For this review, take the finished solid that the model builds, in its own axes (mm). A direction names the side the tool comes from. Round coordinates to 2 decimals unless told otherwise and drop trailing zeros. Write each loop counter-clockwise with the first axis right and the second up, starting at its lowest first coordinate (ties: lowest second). Pieces come first, ordered by that corner, then holes.
from build123d import *

# Parameters (mm, degrees)
SKETCH6_R           = 24
BOSS_EXTRUDE1_DEPTH = 5
SKETCH8_R           = 1.55
CUT_EXTRUDE6_DEPTH  = 5
SKETCH10_R          = 4
BOSS_EXTRUDE2_DEPTH = 36
SKETCH11_R          = 3.5
CUT_EXTRUDE8_DEPTH  = 3


with BuildPart() as part:
    # Sketch6 → Boss-Extrude1 (new body)
    with BuildSketch(Plane.XY):
        Circle(SKETCH6_R)
    extrude(amount=BOSS_EXTRUDE1_DEPTH)

    # Sketch8 → Cut-Extrude6 (cut)
    with BuildSketch(Plane(origin=(0, 0, 0), x_dir=(-1, 0, 0), z_dir=(0, 0, -1))):
        with Locations((0, 20)):
            Circle(SKETCH8_R)
        with Locations((14.142135624, 14.142135624)):
            Circle(SKETCH8_R)
        with Locations((20, 0)):
            Circle(SKETCH8_R)
        with Locations((14.142135624, -14.142135624)):
            Circle(SKETCH8_R)
        with Locations((0, -20)):
            Circle(SKETCH8_R)
        with Locations((-14.142135624, -14.142135624)):
            Circle(SKETCH8_R)
        with Locations((-20, 0)):
            Circle(SKETCH8_R)
        with Locations((-14.142135624, 14.142135624)):
            Circle(SKETCH8_R)
    extrude(amount=-CUT_EXTRUDE6_DEPTH, mode=Mode.SUBTRACT)

    # Sketch10 → Boss-Extrude2 (add)
    with BuildSketch(Plane.XY.offset(5)):
        Circle(SKETCH10_R)
    extrude(amount=BOSS_EXTRUDE2_DEPTH)

    # Sketch11 → Cut-Extrude8 (cut)
    with BuildSketch(Plane.XY.offset(5)):
        with Locations((0, 20)):
            Circle(SKETCH11_R)
        with Locations((14.142135624, 14.142135624)):
            Circle(SKETCH11_R)
        with Locations((20, 0)):
            Circle(SKETCH11_R)
        with Locations((14.142135624, -14.142135624)):
            Circle(SKETCH11_R)
        with Locations((0, -20)):
            Circle(SKETCH11_R)
        with Locations((-14.142135624, -14.142135624)):
            Circle(SKETCH11_R)
        with Locations((-20, 0)):
            Circle(SKETCH11_R)
        with Locations((-14.142135624, 14.142135624)):
            Circle(SKETCH11_R)
    extrude(amount=-CUT_EXTRUDE8_DEPTH, mode=Mode.SUBTRACT)


solid = part.part
(1) We need section A-A, the plane x = 0. Give the boundary of the cut face in (y, z), and give its area (3 significant figures).
Geometry check:
outline: (-24, 0) - (-21.55, 0) - (-21.55, 2) - (-23.5, 2) - (-23.5, 5) - (-24, 5) - close; (-18.45, 0) - (18.45, 0) - (18.45, 2) - (16.5, 2) - (16.5, 5) - (4, 5) - (4, 41) - (-4, 41) - (-4, 5) - (-16.5, 5) - (-16.5, 2) - (-18.45, 2) - close; (21.55, 0) - (24, 0) - (24, 5) - (23.5, 5) - (23.5, 2) - (21.55, 2) - close
area: 474 mm2
(2) For pin 1 Ø5.5 at (x, y) = (-20, 0) entering from -Z; pin 2 Ø10 at (y, z) = (-9, 4) entering from +X; pin 3 Ø3.5 at (x, y) = (-19.5, -1.5) entering from +Z; pin 4 Ø12 at (y, z) = (16, 8) entering from -X, all flat-tipped, find the tip position at first contact; note any pin that passes through.
Geometry check:
pin 1: stops at z = 0
pin 2: stops at x = 23.66
pin 3: stops at z = 2
pin 4: stops at x = -21.43
(3) We need section B-B, the plane y = -20. Give the boundary of the cut face in (x, z), and give its area (3 significant figures).
Geometry check:
outline: (-13.27, 0) - (-1.55, 0) - (-1.55, 2) - (-3.5, 2) - (-3.5, 5) - (-13.27, 5) - close; (1.55, 0) - (13.27, 0) - (13.27, 5) - (3.5, 5) - (3.5, 2) - (1.55, 2) - close
area: 105 mm2
(4) Mouldability with a two-part tool opening along X and no side actions: class faces 3 (the face through (12.71, 13.55, 0.99)), 4 (the face through (-0.867, -3.905, 22.748)), 5 (the face through (0, 0, 41)) as pulls with the +X half, pulls with the -X half, needs draft (parallel to the pull), parting line crosses it, or undercut.
Geometry check:
face 3: undercut
face 4: parting line crosses it
face 5: needs draft
(5) We need section D-D, the plane z = 11.5. Give the boundary of the cut face in (x, y).
Geometry check:
outline: circle Ø8 at (0, 0)
(6) For faces 1 (the face through (-14.98, -12.84, 0.99)), 2 (the face through (16, -15, 2)), list the 3-axis set-ups (+Z, -Z, +X, -X, +Y, -Y) from which the entire face can be reached by the end or side of a thin tool; tool diameter is ignored.
Geometry check:
face 1: +Z, -Z
face 2: +Z
(7) For line 1 along Z through (x, y) = (-12.5, 14.5); line 2 along X through (y, z) = (1.5, 3.5); line 3 along Z through (x, y) = (-15, 10.5), list the stretches that pass through material, from the lowest coordinate up.
Geometry check:
line 1: z = 0 to 2
line 2: x = -23.95 to -23.16, -16.84 to 16.84, 23.16 to 23.95
line 3: z = 0 to 5
